Autodesk Inventor part; units mm, degrees
ref_plane "ANBAU_XY" through (0, 0, 0) normal (-1, 0, 0) x (0, 0, -1)
ref_plane "ANBAU_YZ" through (0, 0, 0) normal (0, 0, -1) x (0, -1, 0)
ref_plane "ANBAU_ZX" through (0, 0, 0) normal (0, -1, 0) x (-1, 0, 0)
sketch "Sketch_11" plane through (0, 0, 0) normal (0, 0, 1) x (1, 0, 0)
  line L0 (0, 0) -> (10, 0)
  line L1 (10, 0) -> (10, 20.5)
  line L2 (10, 20.5) -> (0, 20.5)
  line L3 (0, 20.5) -> (0, 0)
extrude "Extrusion1" add sketch "Sketch_11" along normal mid plane 10
sketch "Sketch2" plane through (0, 0, 5) normal (-1, 0, 0) x (0, 0, 1)
  point P0 (-5, 10.5)
hole "Hole1" at (0, 10.5, 0) direction (1, 0, 0) diameter 3 depth 10
sketch "Sketch_16" plane through (0, 0, 0) normal (0, 0, 1) x (1, 0, 0)
  line L0 (10, 5) -> (0, 5)
  line L1 (0, 5) -> (0, 7)
  line L2 (0, 7) -> (0.379, 6.621)
  line L3 (0.379, 6.621) -> (9.621, 6.621)
  line L4 (9.621, 6.621) -> (10, 7)
  line L5 (10, 7) -> (10, 5)
  line L6 (10, 5) -> (0, 5)
revolve "Revolution1" cut sketch "Sketch_16" angle 360 about axis through (10, 5, 0) along (-1, 0, 0)
thread "Thread1"
sketch "Sketch_17" plane through (0, 0, 0) normal (0, 0, 1) x (1, 0, 0)
  line L0 (10, 16) -> (0, 16)
  line L1 (0, 16) -> (0, 18)
  line L2 (0, 18) -> (0.379, 17.621)
  line L3 (0.379, 17.621) -> (9.621, 17.621)
  line L4 (9.621, 17.621) -> (10, 18)
  line L5 (10, 18) -> (10, 16)
  line L6 (10, 16) -> (0, 16)
revolve "Revolution2" cut sketch "Sketch_17" angle 360 about axis through (10, 16, 0) along (-1, 0, 0)
thread "Thread2"
sketch "Sketch_1" plane through (0, 0, 0) normal (1, 0, 0) x (0, 1, 0)
  arc A0 (-4, 2) -> (-4, -2) centre (-8.5826, 0) ccw
  line L0 (-4, -2) -> (0, -2)
  line L1 (0, -2) -> (0, 2)
  line L2 (0, 2) -> (-4, 2)
extrude "Extrusion2" add sketch "Sketch_1" along normal blind 2.5
ref_plane "ANBAU_XY" through (0, 0, 0) normal (-1, 0, 0) x (0, 0, -1)
ref_plane "ANBAU_YZ" through (0, 0, 0) normal (0, 0, -1) x (0, -1, 0)
ref_plane "ANBAU_ZX" through (0, 0, 0) normal (0, -1, 0) x (-1, 0, 0)
properties part number "HGP-16---(116_JAW)"
The model under review builds one solid part; all positions refer to its coordinate system, in mm. A direction names the side the tool comes from. Round coordinates to 2 decimals unless told otherwise and drop trailing zeros. Order: outer loops, then holes, each group sorted by start corner. A loop starts at its lowest first (then second) coordinate and runs counter-clockwise, first axis right, second up. Notation, with made-up numbers: (6.25, -5) -> (47.25, -5) arc R27 cw to (47.25, 16) -> close; hole circle Ø7 at (43, 46). An arc over 180 degrees is marked (long way). Use CSV: the item, a comma, the result in double quotes. Start each with the question number.
(1) Consider section B-B on x = 2. Write out the cut boundary in (y, z).
(2) Insertion check: pin 1 (3.5 mm diameter, centred on y = 16, z = 0, fed in from -X); pin 2 (1.9 mm diameter, centred on y = 5, z = 0, fed in from -X); pin 3 (1.2 mm diameter, centred on x = 1.5, y = -1.5, fed in from +Z); pin 4 (3 mm diameter, centred on x = 1, y = -3, fed in from -Z). Each pin has a flat end and moves straight along its axis. Give the tip position at first contact, or say it passes through.
(3) Consider section A-A on y = 16. Write out the cut boundary in (x, z).
(4) Wall thickness on probe 1 along Y at (x, z) = (3.75, 0); probe 2 along Z at (x, y) = (2.5, 16); probe 3 along Y at (x, z) = (7.75, -1.25): over which ranges is each line inside the solid? List them lowest first. Write a range as from..to.
(5) Consider section D-D on z = 0. Write out the cut boundary in (x, y).
(6) Consider section C-C on z = -2.75. Write out the cut boundary in (x, y), and give its area (3 significant figures).
(7) Tool access review of faces 5 (the face through (1, -2, -2)), 6 (the face through (2.5, -8, 0)), 7 (the face through (5, 10, 5)): name each direction out of +Z, -Z, +X, -X, +Y, -Y from which nothing blocks a thin tool from reaching the whole face with its end or side.
(8) Mouldability with a two-part tool opening along Z and no side actions: class faces 1 (the face through (5.06, 3.38, 0.07)), 2 (the face through (5, 0, 0)), 3 (the face through (1.23, -13.58, -0.19)), 4 (the face through (1, -2, 2)) as pulls with the +Z half, pulls with the -Z half, needs draft (parallel to the pull), parting line crosses it, or undercut.
Responses:
1,outline,"(-4, -2) -> (0, -2) -> (0, -5) -> (20.5, -5) -> (20.5, 5) -> (0, 5) -> (0, 2) -> (-4, 2) arc R5 ccw (long way) to start; hole circle Ø3.24 at (5, 0); hole circle Ø3 at (10.5, 0); hole circle Ø3.24 at (16, 0)"
2,pin 1,"x = 0.25"
2,pin 2,"through"
2,pin 3,"z = 2"
2,pin 4,"z = -2.89"
3,outline,"(0, -5) -> (10, -5) -> (10, -2) -> (9.62, -1.62) -> (0.38, -1.62) -> (0, -2) -> close; (0, 2) -> (0.38, 1.62) -> (9.62, 1.62) -> (10, 2) -> (10, 5) -> (0, 5) -> close"
4,probe 1,"0..3.38, 6.62..9, 12..14.38, 17.62..20.5"
4,probe 2,"-5..-1.62, 1.62..5"
4,probe 3,"0..3.97, 6.03..9.67, 11.33..14.97, 17.03..20.5"
5,outline,"(0, -13.58) -> (2.5, -13.58) -> (2.5, 0) -> (10, 0) -> (10, 3) -> (9.62, 3.38) -> (0.38, 3.38) -> (0, 3) -> close; (0, 7) -> (0.38, 6.62) -> (9.62, 6.62) -> (10, 7) -> (10, 9) -> (0, 9) -> close; (0, 12) -> (10, 12) -> (10, 14) -> (9.62, 14.38) -> (0.38, 14.38) -> (0, 14) -> close; (0, 18) -> (0.38, 17.62) -> (9.62, 17.62) -> (10, 18) -> (10, 20.5) -> (0, 20.5) -> close"
6,outline,"(0, -12.76) -> (2.5, -12.76) -> (2.5, -4.41) -> (0, -4.41) -> close; (0, 0) -> (10, 0) -> (10, 20.5) -> (0, 20.5) -> close"
6,area,"226 mm²"
7,face 5,"-Z, +X, -X"
7,face 6,"+Z, -Z, +X, -Y"
7,face 7,"+Z, +X, -X, +Y, -Y"
8,face 1,"undercut"
8,face 2,"needs draft"
8,face 3,"parting line crosses it"
8,face 4,"pulls with the +Z half"
